Autodesk Inventor part; units mm, degrees
ref_plane "YZ Plane" through (0, 0, 0) normal (1, 0, 0) x (0, 1, 0)
ref_plane "XZ Plane" through (0, 0, 0) normal (0, 1, 0) x (-1, 0, 0)
ref_plane "XY Plane" through (0, 0, 0) normal (0, 0, 1) x (1, 0, 0)
ref_plane "Work Plane1" through (0, 0, 0) normal (0, 0, 1) x (1, 0, 0)
sketch "Sketch1" plane through (0, 0, 0) normal (0, 0, 1) x (1, 0, 0)
  line L0 (63.5, -8.73) -> (63.5, 39.27)
  line L1 (60.6576, -39.5) -> (69.5, -30.6576)
  line L2 (69.5, -30.6576) -> (69.5, 39.5)
  line L3 (69.5, 39.5) -> (1.55, 39.5)
  line L4 (1.55, 39.5) -> (-11.5, 34.5)
  line L5 (-11.5, 34.5) -> (-67.5, 34.5)
  line L6 (-67.5, 34.5) -> (-69.5, 32.5)
  line L7 (-69.5, 32.5) -> (-69.5, -23.5)
  line L8 (-69.5, -23.5) -> (-67.5, -25.5)
  line L9 (-67.5, -25.5) -> (-11.5, -25.5)
  line L10 (-11.5, -25.5) -> (50.5667, -25.5)
  line L11 (50.5667, -25.5) -> (50.5667, -39.5)
  line L12 (50.5667, -39.5) -> (60.6576, -39.5)
  circle A0 centre (61.5, -3.73) radius 1.6
  circle A1 centre (61.5, 6.27) radius 1.6
  circle A2 centre (61.5, 34.27) radius 1.6
  circle A3 centre (45.5, 34.27) radius 1.6
  circle A4 centre (45.5, 6.27) radius 1.6
  circle A5 centre (45.5, -3.73) radius 1.6
  circle A6 centre (24.65, 15.77) radius 1.6
  circle A7 centre (8.35, 15.77) radius 1.6
  circle A8 centre (-14.5, 4.5) radius 1.95
  circle A9 centre (-39.5, 29.5) radius 1.95
  circle A10 centre (-64.5, -20.5) radius 1.95
  circle A11 centre (-14.5, 29.5) radius 1.95
  circle A12 centre (-64.5, 29.5) radius 1.95
  circle A13 centre (-14.5, -20.5) radius 1.95
  circle A14 centre (-39.5, -20.5) radius 1.95
  circle A15 centre (-64.5, 4.5) radius 1.95
  circle A16 centre (-57, 22) radius 4
  circle A17 centre (-22, -13) radius 4
  circle A18 centre (-57, -13) radius 4
  circle A19 centre (-22, 22) radius 4
  line L13 (70.0555, 39.5) -> (59.0555, 39.5)
  line L14 (59.0555, 39.5) -> (59.0555, 2.5)
  line L15 (59.0555, 2.5) -> (70.0555, 2.5)
  line L16 (70.0555, 2.5) -> (70.0555, 39.5)
  line L17 (70.0555, 39.5) -> (73.0555, 39.5)
  line L18 (73.0555, 39.5) -> (73.0555, 2.5)
  line L19 (73.0555, 2.5) -> (70.0555, 2.5)
  line L20 (70.0555, 2.5) -> (70.0555, 39.5)
  point P0 (0, 0)
  dimension "d0" = 11
  dimension "d1" = 37
  dimension "d2" = 3
extrude "Extrusion1" add sketch "Sketch1" along normal blind 4 contours L15 L14 L3 L2 | L2 L13 L16 L15 | L16 L17 L18 L19
sketch "Sketch2" plane through (73.0555, 2.5, 0) normal (1, 0, 0) x (0, 0, -1)
  circle A0 centre (29, 3.77) radius 1.4
  circle A1 centre (37, 3.77) radius 1.4
  circle A2 centre (21, 3.77) radius 1.4
  circle A3 centre (29, 31.77) radius 1.4
  circle A4 centre (37, 31.77) radius 1.4
  circle A5 centre (21, 31.77) radius 1.4
  circle A6 centre (37, -6.23) radius 1.4
  circle A7 centre (29, -6.23) radius 1.4
  circle A8 centre (21, -6.23) radius 1.4
  line L0 (13, 36.77) -> (45, 36.77)
  line L1 (13, 36.77) -> (13, -11.23)
  line L2 (45, -11.23) -> (13, -11.23)
  line L3 (45, 36.77) -> (45, -11.23)
  line L4 (0, 37) -> (-4, 37)
  line L5 (-4, 37) -> (34, 37)
  line L6 (34, 37) -> (34, 0)
  line L7 (34, 0) -> (-4, 0)
  line L8 (-4, 0) -> (-4, 37)
  point P0 (0, -2.5)
  dimension "d5" = 38
extrude "Extrusion2" add sketch "Sketch2" against normal blind 3.2 contours L1 L7 L8 L4 L5 L6 L0 | L0 L6 L7 L1
properties part number "cellSTORM_Laserrotator_v0"
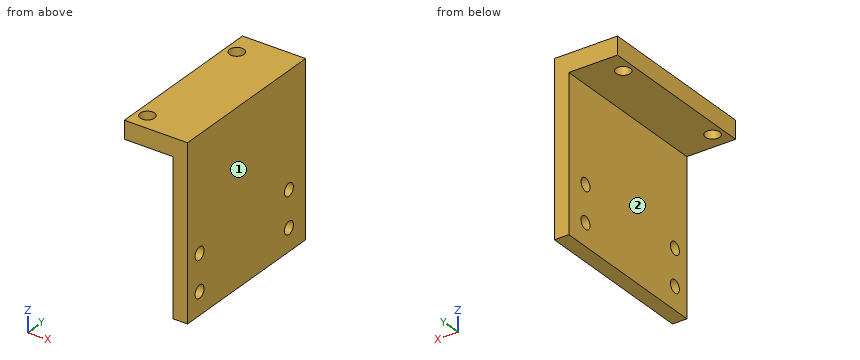
Read the model definition and answer for the solid it produces. Units are mm, in the model's axes. Face numbers are marked on the shaded views. A direction names the side the tool comes from. Coordinates: 2 decimals unless noted, no trailing zeros. Loops run counter-clockwise (first coordinate to the right, second up) from the corner with the lowest first, then second, coordinate; pieces in that order, holes last. Notation, with made-up numbers: (35.25, -37.75) - (51.25, -37.75) arc R16 ccw to (51.25, -7.75) - close; hole circle Ø5 at (-25.75, 48.25). An arc over 180 degrees is marked (long way). Answer in a Markdown table with one row per item.
Q1. Find section D-D on y = 30. Write down the section's boundary in (x, z), plus the area to 3 significant figures.
Here are the results:
| item | result |
|---|---|
| outline | (59.06, 0) - (69.86, 0) - (69.86, -34) - (73.06, -34) - (73.06, 4) - (59.06, 4) - close |
| area | 165 mm^2 |
Q2. Find section C-C on y = 6.27. Write down the section's boundary in (x, z).
Here are the results:
| item | result |
|---|---|
| outline | (59.06, 0) - (59.9, 0) - (59.9, 4) - (59.06, 4) - close; (63.1, 0) - (69.86, 0) - (69.86, -19.6) - (73.06, -19.6) - (73.06, 4) - (63.1, 4) - close; (69.86, -34) - (73.06, -34) - (73.06, -30.4) - (69.86, -30.4) - close; (69.86, -27.6) - (73.06, -27.6) - (73.06, -22.4) - (69.86, -22.4) - close |
Q3. Find section A-A on x = 61.5. Write down the section's boundary in (y, z), plus the area to 3 significant figures.
Here are the results:
| item | result |
|---|---|
| outline | (2.5, 0) - (4.67, 0) - (4.67, 4) - (2.5, 4) - close; (7.87, 0) - (32.67, 0) - (32.67, 4) - (7.87, 4) - close; (35.87, 0) - (39.5, 0) - (39.5, 4) - (35.87, 4) - close |
| area | 122 mm^2 |
Q4. Given P1, Ø5.5, axis at x = 67, y = 21.5, coming from the -Z side; P2, Ø1.7, axis at y = 34.27, z = -29, coming from the -X side; P3, Ø1.5, axis at y = 31, z = -24.5, coming from the -X side, each flat-ended and moving along its own axis, determine where each tip first touches the part or whether it passes through.
Here are the results:
| item | result |
|---|---|
| P1 | stops at z = 0 |
| P2 | passes through |
| P3 | stops at x = 69.86 |
Q5. For the marked faces 1 and 2, determine the directions among +Z, -Z, +X, -X, +Y, -Y from which every point of the face is accessible in a straight line to the end or side of a thin tool.
Here are the results:
| item | result |
|---|---|
| face 1 | +Z, -Z, +X, +Y, -Y |
| face 2 | -Z, -X, +Y, -Y |
Q6. Find section B-B on z = -21. Write down the section's boundary in (x, y).
Here are the results:
| item | result |
|---|---|
| outline | (69.86, 2.5) - (73.06, 2.5) - (73.06, 4.87) - (69.86, 4.87) - close; (69.86, 7.67) - (73.06, 7.67) - (73.06, 32.87) - (69.86, 32.87) - close; (69.86, 35.67) - (73.06, 35.67) - (73.06, 39.5) - (69.86, 39.5) - close |
Q7. Straight lines are drawn through the part: line 1 along Y through (x, z) = (72.35, -29); line 2 along Y through (x, z) = (61.5, 2.35); line 3 along Z through (x, y) = (66.25, 25). For each, find the intervals that lie inside material, in ascending order. Write a range as [from, to].
Here are the results:
| item | result |
|---|---|
| line 1 | y = [2.5, 4.87], [7.67, 32.87], [35.67, 39.5] |
| line 2 | y = [2.5, 4.67], [7.87, 32.67], [35.87, 39.5] |
| line 3 | z = [0, 4] |
